```python
from build123d import *

# Parameters (mm, degrees)
F0_R      = 37.5
F0_R_2    = 35
F1_DEPTH  = 18
F2_R      = 43
F2_R_2    = 35
F3_DEPTH  = 3
F4_R      = 5
F6_R      = 37.5
F6_R_2    = 36.5
F7_DEPTH  = 4.5
F10_DEPTH = 1.5


with BuildPart() as f1:
    # F0 (on Top) → F1 (new body)
    with BuildSketch(Plane.XY):
        Circle(F0_R)
        Circle(F0_R_2, mode=Mode.SUBTRACT)
    extrude(amount=F1_DEPTH)

    # F2 (on Top) → F3 (join)
    with BuildSketch(Plane.XY):
        Circle(F2_R)
        Circle(F2_R_2, mode=Mode.SUBTRACT)
    extrude(amount=F3_DEPTH)

    # F4
    f4_edges = [f1.edges().sort_by_distance(p)[0] for p in [
        (-35, 0, 0),
    ]]
    fillet(f4_edges, radius=F4_R)

    # F6 (on offset) → F7 (cut)
    with BuildSketch(Plane.XY.offset(16)):
        Circle(F6_R)
        Circle(F6_R_2, mode=Mode.SUBTRACT)
    extrude(amount=-F7_DEPTH, mode=Mode.SUBTRACT)

    # F9 (on offset) → F10 (join)
    with BuildSketch(Plane.XY.offset(15)):
        with BuildLine():
            Line((29.580399, 5), (34.641016, 5))
            ThreePointArc((34.641016, 5), (0, 35), (-34.641016, 5))
            Line((-34.641016, 5), (-29.580399, 5))
            ThreePointArc((-29.580399, 5), (0, 30), (29.580399, 5))
        make_face()
        with BuildLine():
            Line((34.641016, -5), (29.580399, -5))
            ThreePointArc((29.580399, -5), (0, -30), (-29.580399, -5))
            Line((-29.580399, -5), (-34.641016, -5))
            ThreePointArc((-34.641016, -5), (0, -35), (34.641016, -5))
        make_face()
    extrude(amount=-F10_DEPTH)


solid = f1.part
```
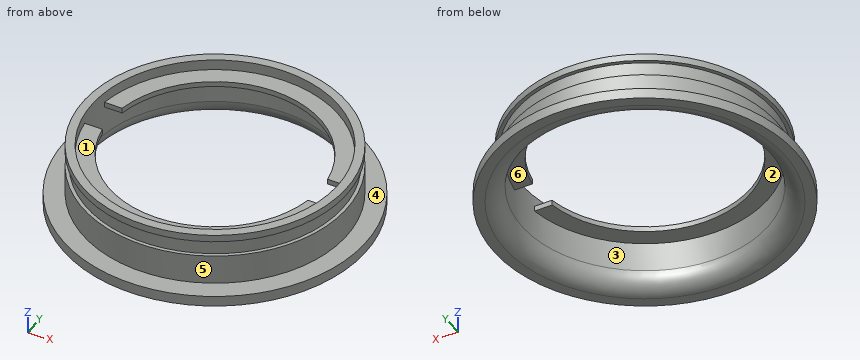
Source: CAD feature listing. Evaluate the final solid. Frame: model axes, mm. Face numbers are marked on the shaded views. A direction names the side the tool comes from. Round coordinates to 2 decimals unless told otherwise and drop trailing zeros. Loops run counter-clockwise (first coordinate to the right, second up) from the corner with the lowest first, then second, coordinate; pieces in that order, holes last. Notation, with made-up numbers: M 46.25,-15 L 89.25,-15 A16 ccw 89.25,16 Z; hole C 21.25,59 d8. An arc over 180 degrees is marked long. Put each result on its own line as item: value.
(1) Section C-C, the plane z = 7. Return loops of the section in (x, y).
Solutions:
outline: C 0,0 d75; hole C 0,0 d70
(2) Section B-B, the plane y = 0. Return loops of the section in (x, z), and give its area (3 significant figures).
Solutions:
outline: M -43,0 L -40,0 A5 ccw -35,5 L -35,18 L -37.5,18 L -37.5,16 L -36.5,16 L -36.5,11.5 L -37.5,11.5 L -37.5,3 L -43,3 Z; M 35,5 A5 ccw 40,0 L 43,0 L 43,3 L 37.5,3 L 37.5,11.5 L 36.5,11.5 L 36.5,16 L 37.5,16 L 37.5,18 L 35,18 Z
area: 103 mm²
(3) Access query for the marked faces 1, 2 and 3. Directions: +Z, -Z, +X, -X, +Y, -Y. A direction counts if a zero-diameter tool reaches every point of the face in a straight line with its end or side. Return the directions, or none.
Solutions:
face 1: +Z
face 2: -Z
face 3: none
(4) First-contact query: pin 1 (1 mm diameter, centred on x = -4.5, z = 4.5, fed in from -Y); pin 2 (1.6 mm diameter, centred on x = -31.5, z = 14.5, fed in from +Y); pin 3 (1.5 mm diameter, centred on x = 13, y = -31.5, fed in from -Z). Flat tips, straight axial feed; report the tip coordinate or a pass-through.
Solutions:
pin 1: y = -37.29
pin 2: y = 19.74
pin 3: z = 13.5
(5) Pull-direction query (Y, two-part tool) for the marked faces 4, 5 and 6; classes: released by +Y, released by -Y, zero draft, split by the parting line, or undercut.
Solutions:
face 4: zero draft
face 5: split by the parting line
face 6: undercut
(6) Ray query, line 1 (Z direction, x = -24, y = 21.5); line 2 (Y direction, x = 0, z = 9.75); line 3 (Y direction, x = -12, z = 6). Return the intervals inside material, ascending. Write a range as [from, to].
Solutions:
line 1: [13.5, 15]
line 2: [-37.5, -35], [35, 37.5]
line 3: [-35.53, -32.88], [32.88, 35.53]
